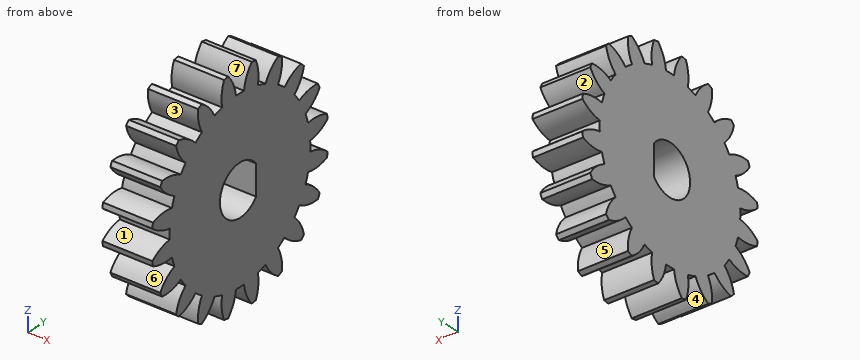
from build123d import *

# Parameters (mm, degrees)
BASPROSKE_W         = 5
BASPROSKE_H         = 11
TOOTHCUT_DEPTH      = 17.340134638
TEETHCUTS_COUNT     = 20
TEETHCUTS_ANGLE     = 342
BORSKE_R            = 1.5
BORE_DEPTH          = 50.0000508
SKETCH1_R           = 2.5
CUT_EXTRUDE1_DEPTH  = 10
SKETCH2_W           = 5.908261021
SKETCH2_H           = 1.397592127
BOSS_EXTRUDE1_DEPTH = 5
SKETCH3_R           = 2.5
CUT_EXTRUDE2_DEPTH  = 10
SKETCH4_W           = 5.744521792
SKETCH4_H           = 0.916677302
BOSS_EXTRUDE2_DEPTH = 5


with BuildPart() as part:
    # BasProSke → Base-Revolve (revolve)
    with BuildSketch(Plane(origin=(0, 0, 0), x_dir=(1, 0, 0), z_dir=(0, 1, 0)), mode=Mode.PRIVATE) as base_revolve_sk:
        with Locations((2.5, 5.5)):
            Rectangle(BASPROSKE_W, BASPROSKE_H)
    revolve(base_revolve_sk.sketch.rotate(Axis((-10, 0, 0), (1, 0, 0)), 180), axis=Axis((-10, 0, 0), (1, 0, 0)))

    # TooCutSke → ToothCut (cut, through all)
    with BuildSketch(Plane(origin=(0, 0, 0), x_dir=(0, 0, -1), z_dir=(1, 0, 0))):
        with BuildLine():
            ThreePointArc((0.499924007, 8.734705318), (0, 8.749), (-0.499924007, 8.734705318))
            ThreePointArc((-0.499924007, 8.734705318), (-0.824302243, 9.905497836), (-1.485192705, 10.924909509))
            ThreePointArc((-1.485192705, 10.924909509), (0, 11.0254), (1.485192705, 10.924909509))
            ThreePointArc((1.485192705, 10.924909509), (0.824302243, 9.905497836), (0.499924007, 8.734705318))
        make_face()
    toothcut = extrude(amount=TOOTHCUT_DEPTH, mode=Mode.SUBTRACT)

    # TeethCuts: ToothCut ×20 about axis
    teethcuts_axis = Axis((-10, 0, 0), (1, 0, 0))
    for i in range(1, TEETHCUTS_COUNT):
        add(toothcut.rotate(teethcuts_axis, i * TEETHCUTS_ANGLE / (TEETHCUTS_COUNT - 1)), mode=Mode.SUBTRACT)

    # BorSke → Bore (cut, symmetric)
    with BuildSketch(Plane(origin=(0, 0, 0), x_dir=(0, 0, -1), z_dir=(1, 0, 0))):
        with Locations(Location((0, 0, 0), (0, 0, 180))):
            Circle(BORSKE_R)
    extrude(amount=BORE_DEPTH, both=True, mode=Mode.SUBTRACT)

    # Sketch1 → Cut-Extrude1 (cut)
    with BuildSketch(Plane(origin=(5, 0, 0), x_dir=(0, 0, -1), z_dir=(1, 0, 0))):
        Circle(SKETCH1_R)
    extrude(amount=-CUT_EXTRUDE1_DEPTH, mode=Mode.SUBTRACT)

    # Sketch2 → Boss-Extrude1 (add)
    with BuildSketch(Plane(origin=(5, 0, 0), x_dir=(0, 0, -1), z_dir=(1, 0, 0))):
        with Locations((-0.183749745, 2.198796064)):
            Rectangle(SKETCH2_W, SKETCH2_H)
    extrude(amount=-BOSS_EXTRUDE1_DEPTH)

    # Sketch3 → Cut-Extrude2 (cut)
    with BuildSketch(Plane.ZY):
        with Locations(Location((0, 0, 0), (0, 0, 180))):
            Circle(SKETCH3_R)
    extrude(amount=-CUT_EXTRUDE2_DEPTH, mode=Mode.SUBTRACT)

    # Sketch4 → Boss-Extrude2 (add, through all)
    with BuildSketch(Plane.ZY):
        with Locations((0.562607804, 2.458338651)):
            Rectangle(SKETCH4_W, SKETCH4_H)
    extrude(amount=-BOSS_EXTRUDE2_DEPTH)


solid = part.part
Work out the finished part from the listing and answer in its coordinate system (mm). Face numbers are marked on the shaded views. A direction names the side the tool comes from. Round coordinates to 2 decimals unless told otherwise and drop trailing zeros. Loops run counter-clockwise (first coordinate to the right, second up) from the corner with the lowest first, then second, coordinate; pieces in that order, holes last. Notation, with made-up numbers: (-31.75, 62.25) - (-8.75, 62.25) arc R29 ccw to (-8.75, 93.25) - close; hole circle Ø3 at (-20.75, -38.5). An arc over 180 degrees is marked (long way). One line per item, written item: value.
Q1. Find section D-D on y = -4.25. Give the vertices of the cut face in (x, z).
Check values:
outline: (0, -9.55) - (5, -9.55) - (5, 9.55) - (0, 9.55) - close
Q2. The mould has two halves that part along Y. Classify the marked faces 1, 2 and 3: +Y half, -Y half, draft (parallel to the pull), parting line (faces both ways), or undercut.
Check values:
face 1: -Y half
face 2: +Y half
face 3: undercut
Q3. Each of these flat-tipped pins is pushed along its axis until it touches: pin 1 Ø3 at (x, z) = (2, 6) entering from +Y; pin 2 Ø2.5 at (x, z) = (2.5, 0) entering from -Y; pin 3 Ø1 at (x, y) = (4, -4) entering from -Z. Where does it stop, or does it pass through?
Check values:
pin 1: y = 9.92
pin 2: y = -10.63
pin 3: z = -9.75
Q4. Straight lines are drawn through the part: probe 1 along Y at (x, z) = (2.7, 0); probe 2 along Z at (x, y) = (2.2, 0); probe 3 along Z at (x, y) = (1.85, 7.25). For each, find the intervals that lie inside material, in ascending order.
Check values:
probe 1: -8.75 to -2.5, 2 to 8.75
probe 2: -8.75 to -2.5, 2.5 to 8.75
probe 3: -7.86 to -6.07, -4.9 to 4.9, 6.07 to 7.86
Q5. Find section A-A on y = 0. Give the vertices of the cut face in (x, z), and give its area (3 significant figures).
Check values:
outline: (0, -8.75) - (5, -8.75) - (5, -2.5) - (0, -2.5) - close; (0, 2.5) - (5, 2.5) - (5, 8.75) - (0, 8.75) - close
area: 62.5 mm2
Q6. Find section B-B on z = 0. Give the vertices of the cut face in (x, y).
Check values:
outline: (0, -8.75) - (5, -8.75) - (5, -2.5) - (0, -2.5) - close; (0, 2) - (5, 2) - (5, 8.75) - (0, 8.75) - close
Q7. Find section C-C on z = -9. Give the vertices of the cut face in (x, y).
Check values:
outline: (0, -5.23) - (5, -5.23) - (5, -3.7) - (0, -3.7) - close; (0, -2.29) - (5, -2.29) - (5, -0.54) - (0, -0.54) - close; (0, 0.54) - (5, 0.54) - (5, 2.29) - (0, 2.29) - close; (0, 3.7) - (5, 3.7) - (5, 5.23) - (0, 5.23) - close
Q8. For the marked faces 4, 5, 6 and 7, determine the directions among +Z, -Z, +X, -X, +Y, -Y from which every point of the face is accessible in a straight line to the end or side of a thin tool.
Check values:
face 4: -Z, +X, -X
face 5: +X, -X
face 6: +X, -X, -Y
face 7: +Z, +X, -X
